```python
from build123d import *

# Parameters (mm, degrees)
SKETCH_1_W               = 72.5
SKETCH_1_H               = 50
EXTRUDE_1_DEPTH          = 4
SHELL_1_T                = 1.8
CUT_EXTRUDE_1_DEPTH      = 48.157210477
CUT_EXTRUDE_1_DEPTH_BACK = 4


with BuildPart() as part:
    # 草图1 → 凸台-拉伸1 (new body)
    with BuildSketch(Plane.XY):
        Rectangle(SKETCH_1_W, SKETCH_1_H)
    extrude(amount=EXTRUDE_1_DEPTH)

    # 抽壳1
    shell_1_openings = [part.faces().sort_by_distance(p)[0] for p in [
        (36.25, 0, 2),
    ]]
    offset(amount=SHELL_1_T, openings=shell_1_openings, kind=Kind.INTERSECTION)

    # 草图2 → 切除-拉伸1 (cut, two sides: drawn at the far end of the back side and taken through both)
    with BuildSketch(Plane.XY.offset(5.8).offset(-CUT_EXTRUDE_1_DEPTH_BACK)):
        Polygon((34.25, 23), (36.25, 23), (36.25, -23), (34.25, -23), (-34.25, -23), (-34.25, 23), align=None)
    extrude(amount=CUT_EXTRUDE_1_DEPTH + CUT_EXTRUDE_1_DEPTH_BACK, mode=Mode.SUBTRACT)


solid = part.part
```
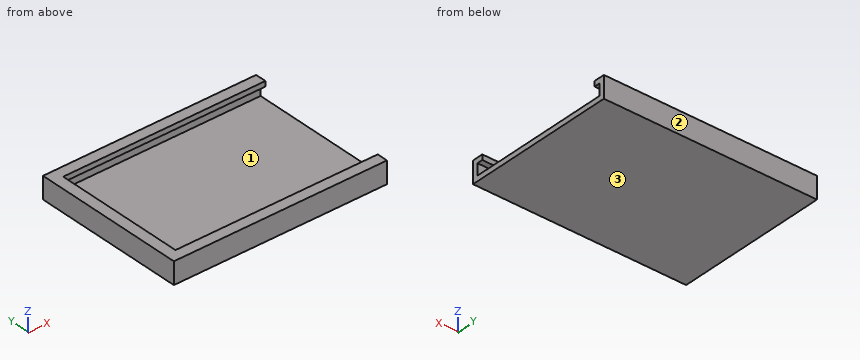
Build history of the part. All positions in model axes, mm. Face numbers are marked on the shaded views. Give positions to 0.01 mm unless a question says otherwise; leave off trailing zeros. Loops run counter-clockwise (first coordinate to the right, second up) from the corner with the lowest first, then second, coordinate; pieces in that order, holes last.
1) Drop flat-ended pins along their axis: P1, Ø2, axis at x = 5, y = 6.5, coming from the +Z side; P2, Ø2, axis at y = -1.5, z = 5, coming from the +X side. Give the stop position or say it passes through.
Values follow:
P1: stops at z = 0
P2: stops at x = -34.25
2) Two-plate mould, pull along Y, no slides. Class the marked faces 1, 2 and 3: released by +Y, released by -Y, zero draft, split by the parting line, or undercut.
Values follow:
face 1: undercut
face 2: released by +Y
face 3: zero draft
3) Band-saw the part on A-A on x = -8. List the corners of the cut face in (y, z), then the cut area to 3 significant figures.
Values follow:
outline: (-26.8, -1.8) - (26.8, -1.8) - (26.8, 5.8) - (23, 5.8) - (23, 4) - (25, 4) - (25, 0) - (-25, 0) - (-25, 4) - (-23, 4) - (-23, 5.8) - (-26.8, 5.8) - close
area: 125 mm2
4) Band-saw the part on B-B on y = -16. List the corners of the cut face in (x, z).
Values follow:
outline: (-38.05, -1.8) - (36.25, -1.8) - (36.25, 0) - (-36.25, 0) - (-36.25, 4) - (-34.25, 4) - (-34.25, 5.8) - (-38.05, 5.8) - close
5) Probe line 1 along Y through (x, z) = (-30.5, 5.5); line 2 along Z through (x, y) = (-15.5, -23.5); line 3 along Y through (x, z) = (5.5, 0.25). List the from-to ranges inside material, lowest first.
Values follow:
line 1: y = -26.8 to -23, 23 to 26.8
line 2: z = -1.8 to 0, 4 to 5.8
line 3: y = -26.8 to -25, 25 to 26.8
6) Band-saw the part on C-C on z = 5. List the corners of the cut face in (x, y).
Values follow:
outline: (-38.05, -26.8) - (36.25, -26.8) - (36.25, -23) - (-34.25, -23) - (-34.25, 23) - (36.25, 23) - (36.25, 26.8) - (-38.05, 26.8) - close
